Can you work these out from the model? Positions are in its coordinate system, mm. Face numbers are marked on the shaded views. A direction names the side the tool comes from. Coordinates: 2 decimals unless noted, no trailing zeros. Order: outer loops, then holes, each group sorted by start corner. A loop starts at its lowest first (then second) coordinate and runs counter-clockwise, first axis right, second up. Notation, with made-up numbers: (-14.75, 63) -> (2.25, 63) arc R9 ccw to (2.25, 71) -> close; hole circle Ø7 at (-29.75, -36). An arc over 180 degrees is marked (long way). Answer as a JSON object with one key per item and string values. Group by question number.
(1) I want a section at D-D, the plane z = 32.5. List the corners of the cut face in (x, y) for me, plus the area to 3 significant figures.
(2) Which directions (+Z, -Z, +X, -X, +Y, -Y) give clear straight access to the entire face, cutting with the end or side of a thin tool? Please do the marked faces 5, 6 and 7.
(3) I need wall thicknesses on line 1 (X direction, y = -36, z = 8); line 2 (X direction, y = -71, z = 50); line 3 (Z direction, x = 42, y = -42.3). Which ranges of each line are inside material? Lowest first, please.
(4) I want a section at B-B, the plane z = 75. List the corners of the cut face in (x, y) for me, plus the area to 3 significant figures.
(5) I want a section at A-A, the plane y = -8.5. List the corners of the cut face in (x, z) for me, plus the area to 3 significant figures.
(6) If we mould it in two halves opening along X, with no side actions, what happens to the marked faces 1, 2, 3 and 4? For each: pulls with the +X half, pulls with the -X half, needs draft (parallel to the pull), parting line crosses it, or undercut.
(7) For pin 1 (3 mm diameter, centred on x = 2.5, z = 65.5, fed in from -Y); pin 2 (3 mm diameter, centred on x = 38, z = 78, fed in from +Y); pin 3 (3 mm diameter, centred on y = 44.5, z = 16.5, fed in from -X), each with a flat end and sliding along its axis, tell me the tip position at first contact or that it passes through.
(8) I want a section at C-C, the plane y = -79. List the corners of the cut face in (x, z) for me.
Autodesk Inventor part; units mm, degrees
ref_plane "YZ Plane" through (0, 0, 0) normal (1, 0, 0) x (0, 1, 0)
ref_plane "XZ Plane" through (0, 0, 0) normal (0, 1, 0) x (-1, 0, 0)
ref_plane "XY Plane" through (0, 0, 0) normal (0, 0, 1) x (1, 0, 0)
sketch "Boceto1" plane through (0, 0, 0) normal (0, 0, 1) x (1, 0, 0)
  line L0 (-40, 75) -> (40, 75)
  line L1 (40, 75) -> (40, -75)
  line L2 (40, -75) -> (-40, -75)
  line L3 (-40, -75) -> (-40, 75)
  line L4 (-40, 75) -> (40, -75) construction
  line L5 (40, 75) -> (-40, -75) construction
  line L6 (37.5, 72.5) -> (-37.5, 72.5)
  line L7 (-37.5, 72.5) -> (-37.5, -74.5)
  line L8 (-37.5, -74.5) -> (37.5, -74.5)
  line L9 (37.5, -74.5) -> (37.5, 72.5)
  point P0 (0, 0)
  dimension "d0" = 80
  dimension "d1" = 150
  dimension "d2" = 2.5
  dimension "d32" = 0.5
extrude "Extrusión1" add sketch "Boceto1" along normal blind 50
extrude "Extrusión2" add sketch "Boceto1" along normal blind 0.5 contours L9 L8 L7 L6
sketch "Boceto2" plane through (40, -75, 0) normal (1, 0, 0) x (0, 0, -1)
  circle A0 centre (-75, 14.3207) radius 32.5
  line L0 (-106.2586, 14.1414) -> (-42.2586, 14.1414) construction
  line L1 (0, 0) -> (-50, 0)
  line L2 (-87, 2.3207) -> (-63, 2.3207)
  line L3 (-63, 2.3207) -> (-63, 32.3207)
  line L4 (-63, 32.3207) -> (-87, 32.3207)
  line L5 (-87, 32.3207) -> (-87, 2.3207)
  line L6 (-0.5, 0.5) -> (-50, 0.5)
  line L7 (0, 150) -> (0, 0)
  line L8 (-49.75, 14.1414) -> (25.25, 14.1414) construction
  point P0 (0, 75)
  dimension "d9" = 65
  dimension "d15" = 24
  dimension "d16" = 30
extrude "Extrusión3" cut sketch "Boceto2" against normal blind 10 contours L5 L4 L3 L2
extrude "Extrusión4" add sketch "Boceto2" along normal blind 25 contours A0 | L5 L4 L3 L2
mirror "Simetría1" about plane through (0, 0, 0) normal (1, 0, 0) of "Extrusión4", "Extrusión3"
sketch "Boceto3" plane through (40, -75, 0) normal (0, -1, 0) x (1, 0, 0)
  line L0 (-80, 0) -> (-80, 50)
  line L1 (-2.5, 0.5) -> (-2.5, 50)
  line L2 (-80, 107.5) -> (-80, 45.8252)
  line L3 (-80, 50) -> (-80, 100)
  line L4 (-80, 100) -> (0, 100)
  line L5 (0, 0) -> (0, 50)
  line L6 (0, 100) -> (0, 50)
  line L7 (0, 50) -> (-2.5, 50)
  line L8 (-2.5, 50) -> (-2.5, 97.5)
  line L9 (-2.5, 97.5) -> (-77.5, 97.5)
  line L10 (-77.5, 97.5) -> (-77.5, 50)
  line L11 (-77.5, 50) -> (-80, 50)
  line L12 (-77.5, 50) -> (-2.5, 50)
  line L13 (-77.5, 50) -> (-2.5, 50)
  point P0 (-40, 0)
  dimension "d24" = 50
  dimension "d25" = 80
  dimension "d26" = 47.5
  dimension "d27" = 75
extrude "Extrusión5" add sketch "Boceto3" against normal blind 70 contours L4 L6 L7 L8 L9 L10 L11 L2
extrude "Extrusión6" add sketch "Boceto3" against normal blind 0.5 contours L10 L9 L8 L12
extrude "Extrusión7" cut sketch "Boceto2" against normal blind 80 contours L5 L4 L3 L2
ref_plane "Plano de trabajo1" through (-40, -93.1793, 75) normal (0, -1, 0) x (1, 0, 0)
sketch "Boceto4" plane through (40, -75, 0) normal (1, 0, 0) x (0, 0, -1)
  line L0 (0, 0) -> (0, 150)
  line L1 (21.5, -18.1793) -> (-129, -18.1793)
  line L2 (-12, 31.3207) -> (-12, 131.3207) construction
  line L3 (-21.5167, 81.3207) -> (7.9238, 81.3207)
  line L4 (-0.5, 147.5) -> (-0.5, 0.5)
  line L5 (-8, 131.3207) -> (-8, 121.3207)
  line L6 (-8.9804, 121.3207) -> (-14.9804, 121.3207)
  line L7 (-14.9804, 121.3207) -> (-14.9804, 101.3207)
  line L8 (-14.9804, 101.3207) -> (-8.9804, 101.3207)
  line L9 (-8.9804, 101.3207) -> (-8.9804, 121.3207)
  line L10 (-11, 101.3207) -> (-11, 103.5079)
  point P0 (0, 75)
  dimension "d39" = 100
  dimension "d45" = 24
  dimension "d46" = 10
  dimension "d47" = 8
  dimension "d49" = 20
  dimension "d53" = 6
ref_plane "Plano de trabajo2" through (40, 56.3207, 12) normal (0, 1, 0) x (-1, 0, 0)
sketch "Boceto5" plane through (40, 56.3207, 12) normal (0, 1, 0) x (-1, 0, 0)
  line L0 (0, 0) -> (-2, 0)
  circle A0 centre (-2, 0) radius 2
  arc A1 (0, 2.2361) -> (0, -2.2361) centre (-2, 0) ccw
  line L1 (0, -2.2361) -> (0, 2.2361)
  point P0 (40, -12)
  dimension "d40" = 2
  dimension "d41" = 6
extrude "Extrusión8" add sketch "Boceto5" against normal blind 5
ref_plane "Plano de trabajo3" through (40, 6.3207, 21.5167) normal (0, -1, 0) x (0, 0, -1)
mirror "Simetría2" about plane through (40, 6.3207, 21.5167) normal (0, -1, 0) of "Extrusión8"
extrude "Extrusión9" cut sketch "Boceto4" against normal through all
ref_plane "Plano de trabajo4" through (0, -75, 0) normal (1, 0, 0) x (0, 0, -1)
mirror "Simetría3" about plane through (0, -75, 0) normal (1, 0, 0) of "Extrusión8", "Simetría2"
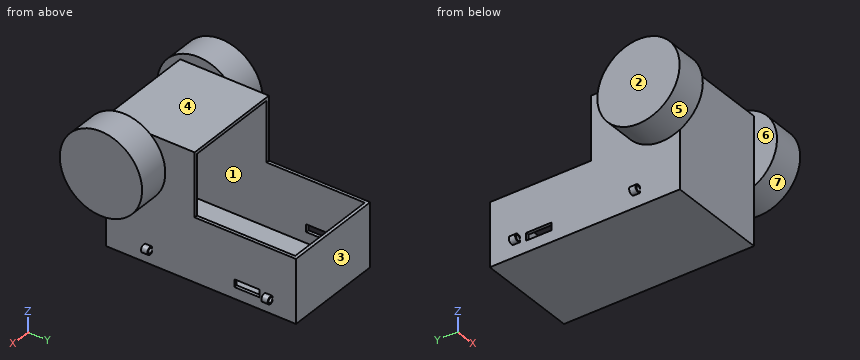
Computed values:
{
 "1": {"outline": "(-40, -75) -> (40, -75) -> (40, 75) -> (-40, 75) -> close; hole (-37.5, -74.5) -> (37.5, -74.5) -> (37.5, 72.5) -> (-37.5, 72.5) -> close", "area": "975 mm2"},
 "2": {"face 5": "-X", "face 6": "+Z, -Y", "face 7": "+X"},
 "3": {"line 1": "x = -40 to -37.5, 37.5 to 40", "line 2": "x = -65 to -37.5, 37.5 to 65", "line 3": "z = 9 to 10, 14 to 15, 48.2 to 101.8"},
 "4": {"outline": "(-65, -93.18) -> (-40, -93.18) -> (-40, -75) -> (40, -75) -> (40, -93.18) -> (65, -93.18) -> (65, -28.18) -> (40, -28.18) -> (40, -5) -> (37.5, -5) -> (37.5, -42.68) -> (40, -42.68) -> (40, -72.68) -> (37.5, -72.68) -> (37.5, -74.5) -> (-37.5, -74.5) -> (-37.5, -72.68) -> (-40, -72.68) -> (-40, -42.68) -> (-37.5, -42.68) -> (-37.5, -5) -> (-40, -5) -> (-40, -28.18) -> (-65, -28.18) -> close", "area": "3,490 mm2"},
 "5": {"outline": "(-40, 0) -> (40, 0) -> (40, 100) -> (-40, 100) -> close; hole (-37.5, 0.5) -> (37.5, 0.5) -> (37.5, 97.5) -> (-37.5, 97.5) -> close", "area": "725 mm2"},
 "6": {"face 1": "undercut", "face 2": "pulls with the -X half", "face 3": "needs draft", "face 4": "undercut"},
 "7": {"pin 1": "stops at y = -75", "pin 2": "stops at y = -5", "pin 3": "stops at x = -40"},
 "8": {"outline": "(-65, 48.16) -> (-40, 48.16) -> (-40, 101.84) -> (-65, 101.84) -> close; (40, 48.16) -> (65, 48.16) -> (65, 101.84) -> (40, 101.84) -> close"}
}
